Geometry: final body of the model. Coordinates: model frame, mm. A direction names the side the tool comes from. Give positions to 0.01 mm unless a question says otherwise; leave off trailing zeros. Order: outer loops, then holes, each group sorted by start corner. A loop starts at its lowest first (then second) coordinate and runs counter-clockwise, first axis right, second up. Notation, with made-up numbers: (59, 7.5) - (106, 7.5) arc R28 cw to (106, 35.5) - close; hole circle Ø5 at (89.25, 65.25). An arc over 180 degrees is marked (long way). One line per question, with ' | ' between items. Start each with the question number.
from build123d import *

# Parameters (mm, degrees)
SKETCH1_W           = 50
SKETCH1_H           = 50
BOSS_EXTRUDE1_DEPTH = 200
SKETCH2_W           = 6
SKETCH2_H           = 50
BOSS_EXTRUDE2_DEPTH = 50
SKETCH4_W           = 20
SKETCH4_H           = 6
CUT_EXTRUDE1_DEPTH  = 2
SKETCH5_W           = 11.315
SKETCH5_H           = 6.095
CUT_EXTRUDE2_DEPTH  = 10.84


with BuildPart() as part:
    # Sketch1 → Boss-Extrude1 (new body)
    with BuildSketch(Plane.XY):
        with Locations((25, -25)):
            Rectangle(SKETCH1_W, SKETCH1_H)
    extrude(amount=BOSS_EXTRUDE1_DEPTH)

    # Sketch2 → Boss-Extrude2 (add)
    with BuildSketch(Plane.XY.offset(200)):
        with Locations((3, -25)):
            Rectangle(SKETCH2_W, SKETCH2_H)
    extrude(amount=BOSS_EXTRUDE2_DEPTH)

    # Sketch4 → Cut-Extrude1 (cut)
    with BuildSketch(Plane(origin=(6, 0, 0), x_dir=(0, 0, -1), z_dir=(1, 0, 0))):
        with Locations((-235, -23)):
            Rectangle(SKETCH4_W, SKETCH4_H)
    extrude(amount=-CUT_EXTRUDE1_DEPTH, mode=Mode.SUBTRACT)

    # Sketch5 → Cut-Extrude2 (cut)
    with BuildSketch(Plane(origin=(0, 0, 0), x_dir=(-1, 0, 0), z_dir=(0, 0, -1))):
        Polygon((-36.315, -18.905), (-36.315, -25), (-25, -25), (-13.685, -25), (-13.685, -18.905), align=None)
        with Locations((-30.6575, -28.0475)):
            Rectangle(SKETCH5_W, SKETCH5_H)
        with Locations((-19.3425, -28.0475)):
            Rectangle(SKETCH5_W, SKETCH5_H)
    extrude(amount=-CUT_EXTRUDE2_DEPTH, mode=Mode.SUBTRACT)


solid = part.part
(1) Cut plane B-B, the plane y = -41. Return the cut outline in (x, z), plus the area to 3 significant figures.
(2) Cut plane C-C, the plane x = 40.5. Return the cut outline in (y, z).
(3) Pull-direction query (Y, two-part tool) for faces 4 (the flat face through (25, 0, 95)), 5 (the flat face through (36.315, -25, 5)), 6 (the flat face through (50, -25, 99)); classes: +Y half, -Y half, draft (parallel to the pull), parting line (faces both ways), or undercut.
(4) Material intervals for line 1 along Z through (x, y) = (8.5, -16); line 2 along X through (y, z) = (-6, 204.5); line 3 along Z through (x, y) = (24, -22), sorted ascending. Write a range as from..to.
(5) Access query for faces 1 (the flat face through (6, -25.3, 224.6)), 2 (the flat face through (25, -31.095, 5)), 3 (the flat face through (4, -23, 235)). Directions: +Z, -Z, +X, -X, +Y, -Y. A direction counts if a zero-diameter tool reaches every point of the face in a straight line with its end or side. Return the directions, or none.
(6) Contact query for flat-ended pins moving along their axis: P1, Ø6.5, axis at y = -23, z = 231.5, coming from the +X side; P2, Ø2, axis at x = 20, y = -23, coming from the +Z side. Output: stop coordinate, or through.
(7) Cut plane A-A, the plane x = 26. Return the cut outline in (y, z) (3 decimals).
Results are:
1) outline: (0, 0) - (50, 0) - (50, 200) - (6, 200) - (6, 250) - (0, 250) - close | area: 10,300 mm2
2) outline: (-50, 0) - (0, 0) - (0, 200) - (-50, 200) - close
3) face 4: +Y half | face 5: undercut | face 6: draft
4) line 1: 0..200 | line 2: 0..6 | line 3: 10.84..200
5) face 1: +Z, +X, +Y, -Y | face 2: -Z | face 3: +X
6) P1: x = 6 | P2: z = 200
7) outline: (-50, 0) - (-31.095, 0) - (-31.095, 10.84) - (-18.905, 10.84) - (-18.905, 0) - (0, 0) - (0, 200) - (-50, 200) - close
